CAD build for the part. Positions are in the model's coordinates, mm. Give positions to 0.01 mm unless a question says otherwise; leave off trailing zeros. Write each loop counter-clockwise with the first axis right and the second up, starting at its lowest first coordinate (ties: lowest second). Pieces come first, ordered by that corner, then holes. Notation, with made-up numbers: (-12, 55) -> (43, 55) arc R37 cw to (43, 93) -> close; hole circle Ø3 at (18.5, 57). An arc over 180 degrees is marked (long way). Use one line per item in the form item = value. Start each with the question number.
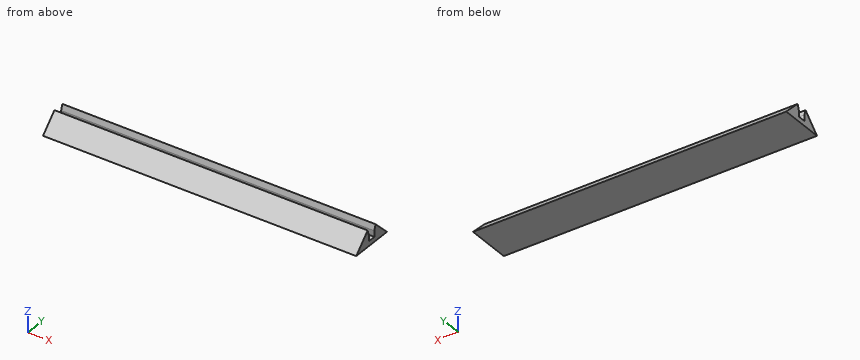
Autodesk Fusion 360 part; units mm, degrees
sketch "Esquisse1" plane through (0, 0, 0) normal (1, 0, 0) x (0, 1, 0)
  line L0 (0, 0) -> (9.15, 0)
  line L1 (9.15, 0) -> (1.65, 7.5)
  line L2 (1.65, 7.5) -> (1.65, 2)
  line L3 (1.65, 2) -> (0, 2)
  line L4 (0, 2.5) -> (0, 20)
  line L5 (-1.65, 2) -> (0, 2)
  line L6 (0, 0) -> (-9.15, 0)
  line L7 (-1.65, 7.5) -> (-1.65, 2)
  line L8 (-9.15, 0) -> (-1.65, 7.5)
  dimension "d2" = 45
  dimension "d3" = 5.5
  dimension "d5" = 2
  dimension "d6" = 3.3
extrude "Extrusion1" add sketch "Esquisse1" along normal blind 130
chamfer "Chanfrein1" distance 3 distance2 1 1 edges at (65, -1.65, 7.5) measured on face at (43.3333, -1.65, 5.6667)
chamfer "Chanfrein2" distance 1 distance2 3 1 edges at (65, 1.65, 7.5) measured on face at (43.3333, 6.65, 2.5)
component "Component" placed x (1, 0, 0) y (0, 1, 0) z (0, 0, 1) at (0, 0, 0)
1) Cut at D-D (y = 7). Give the cut face in (x, z), and give its area (4 significant figures).
2) Cut at A-A (z = 5.75). Give the cut face in (x, y), and give its area (3 significant figures).
3) Cut at B-B (x = 67). Give the cut face in (y, z), and give its area (3 significant figures).
4) Pin check, flat tips, straight feed: pin 1 (3 mm diameter, centred on x = 109, y = 7, fed in from +Z); pin 2 (5 mm diameter, centred on x = 70, y = -3, fed in from +Z); pin 3 (0.8 mm diameter, centred on x = 36, z = 3, fed in from +Y). Stop position of each tip, or through.
5) Wall check: line 1 along Z through (x, y) = (83, -0.75); line 2 along Y through (x, z) = (107.5, 5); line 3 along Z through (x, y) = (9.5, 7.5). Give the ranges that are in metal, low to high. Write a range as from..to.
6) Cut at C-C (y = -6.5). Give the cut face in (x, z), and give its area (4 significant figures).
Final values:
q1.outline = (0, 0) -> (130, 0) -> (130, 2.15) -> (0, 2.15) -> close
q1.area = 279.5 mm^2
q2.outline = (0, -3.4) -> (130, -3.4) -> (130, -2.04) -> (0, -2.04) -> close; (0, 2.04) -> (130, 2.04) -> (130, 3.4) -> (0, 3.4) -> close
q2.area = 355 mm^2
q3.outline = (-9.15, 0) -> (9.15, 0) -> (2.36, 6.79) -> (1.65, 4.5) -> (1.65, 2) -> (-1.65, 2) -> (-1.65, 4.5) -> (-2.36, 6.79) -> close
q3.area = 60.7 mm^2
q4.pin_1 = 3.65
q4.pin_2 = 6.79
q4.pin_3 = 6.55
q5.line_1 = 0..2
q5.line_2 = -4.15..-1.8, 1.8..4.15
q5.line_3 = 0..1.65
q6.outline = (0, 0) -> (130, 0) -> (130, 2.65) -> (0, 2.65) -> close
q6.area = 344.5 mm^2
